from build123d import *

# Parameters (mm, degrees)
F0_W     = 812.8
F0_H     = 812.8
F1_DEPTH = 279.4
F2_W     = 762
F2_H     = 711.2
F3_DEPTH = 254
F4_W     = 25.4
F4_H     = 25.4
F5_DEPTH = 50.8
F6_W     = 228.6
F6_H     = 25.4
F6_W_2   = 25.4
F7_DEPTH = 25.4
F8_W     = 762
F8_H     = 50.8
F9_DEPTH = 254


with BuildPart() as f1:
    # F0 (on Top) → F1 (new body)
    with BuildSketch(Plane.XY):
        with Locations((406.4, 406.4)):
            Rectangle(F0_W, F0_H)
    extrude(amount=F1_DEPTH)

    # F2 (on face) → F3 (cut)
    with BuildSketch(Plane.XY.offset(279.4)):
        with Locations((406.4, 381)):
            Rectangle(F2_W, F2_H)
    extrude(amount=-F3_DEPTH, mode=Mode.SUBTRACT)

    # F4 (on face) → F5 (join)
    with BuildSketch(Plane.YZ.offset(812.8)):
        with Locations((292.1, 139.7)):
            Rectangle(F4_W, F4_H)
        with Locations((520.7, 139.7)):
            Rectangle(F4_W, F4_H)
    extrude(amount=F5_DEPTH)

    # F6 (on face) → F7 (join)
    with BuildSketch(Plane.YZ.offset(863.6)):
        with Locations((419.1, 139.7)):
            Rectangle(F6_W, F6_H)
        with Locations((292.1, 139.7)):
            Rectangle(F6_W_2, F6_H)
    extrude(amount=F7_DEPTH)

    # F8 (on face) → F9 (cut)
    with BuildSketch(Plane.XY.offset(279.4)):
        with Locations((406.4, 762)):
            Rectangle(F8_W, F8_H)
    extrude(amount=-F9_DEPTH, mode=Mode.SUBTRACT)


solid = f1.part
Input: part model. Units: mm. Frame: model coordinates. A direction names the side the tool comes from. Coordinates: 2 decimals unless noted, no trailing zeros. Order: outer loops, then holes, each group sorted by start corner. A loop starts at its lowest first (then second) coordinate and runs counter-clockwise, first axis right, second up. Notation, with made-up numbers: M 1,63 L 45,63 A4 cw 45,68 Z; hole C 59.5,-3 d3. An arc over 180 degrees is marked long. Write item = value, one per line. Start each with the question number.
(1) Pull-direction query (Y, two-part tool) for faces 6 (the flat face through (838, 508, 140)), 7 (the flat face through (401, 0, 138)), 8 (the flat face through (863.6, 405, 140)), 9 (the flat face through (0, 401, 138)); classes: released by +Y, released by -Y, zero draft, split by the parting line, or undercut.
(2) Section C-C on x = 665. Output: boundary loops of the cut face in (y, z).
(3) Section A-A on y = 354. Output: boundary loops of the cut face in (x, z), and give its area (3 significant figures).
(4) First-contact query: P1, Ø7.5, axis at x = 829.5, z = 137.5, coming from the -Y side; P2, Ø10, axis at y = 586.5, z = 214.5, coming from the +X side; P3, Ø20.5, axis at x = 868, z = 137.5, coming from the +Y side. Flat tips, straight axial feed; report the tip coordinate or a pass-through.
(5) Section B-B on z = 98. Output: boundary loops of the cut face in (x, y), and give its area (3 significant figures).
(6) Line query: line 1 along Y through (x, z) = (331, 182); line 2 along Z through (x, y) = (303.5, 672). Output: solid intervals per line, ascending. Write a range as [from, to].
(7) Reachability of faces 1 (the flat face through (867, 405, 127)), 2 (the flat face through (850, 279.4, 140)), 3 (the flat face through (867, 408, 152.4)), 4 (the flat face through (401, 412, 25.4)), 5 (the flat face through (838, 304.8, 140)) from +Z, -Z, +X, -X, +Y, -Y: full face, straight path, thin tool, end or side. Return the list, or none.
Result set:
q1.face_6 = undercut
q1.face_7 = released by -Y
q1.face_8 = undercut
q1.face_9 = zero draft
q2.outline = M 0,0 L 812.8,0 L 812.8,279.4 L 787.4,279.4 L 787.4,25.4 L 25.4,25.4 L 25.4,279.4 L 0,279.4 Z
q3.outline = M 0,0 L 812.8,0 L 812.8,279.4 L 787.4,279.4 L 787.4,25.4 L 25.4,25.4 L 25.4,279.4 L 0,279.4 Z; M 863.6,127 L 889,127 L 889,152.4 L 863.6,152.4 Z
q3.area = 34,200 mm²
q4.P1 = 279.4
q4.P2 = 812.8
q4.P3 = 533.4
q5.outline = M 0,0 L 812.8,0 L 812.8,812.8 L 0,812.8 Z; hole M 25.4,25.4 L 787.4,25.4 L 787.4,787.4 L 25.4,787.4 Z
q5.area = 80,000 mm²
q6.line_1 = [0, 25.4], [787.4, 812.8]
q6.line_2 = [0, 25.4]
q7.face_1 = -Z, +X, +Y, -Y
q7.face_2 = +Z, -Z, +X, -Y
q7.face_3 = +Z, +X, +Y, -Y
q7.face_4 = +Z
q7.face_5 = +Z, -Z
